Model file for the job. Use its own axes, mm. Face numbers are marked on the shaded views. Round coordinates to 2 decimals unless told otherwise and drop trailing zeros. Write each loop counter-clockwise with the first axis right and the second up, starting at its lowest first coordinate (ties: lowest second). Pieces come first, ordered by that corner, then holes. Notation, with made-up numbers: (38.25, 85.25) - (48.25, 85.25) arc R14 ccw to (48.25, 99.25) - close; hole circle Ø7 at (71.5, 2.25). An arc over 180 degrees is marked (long way). One line per item, written item: value.
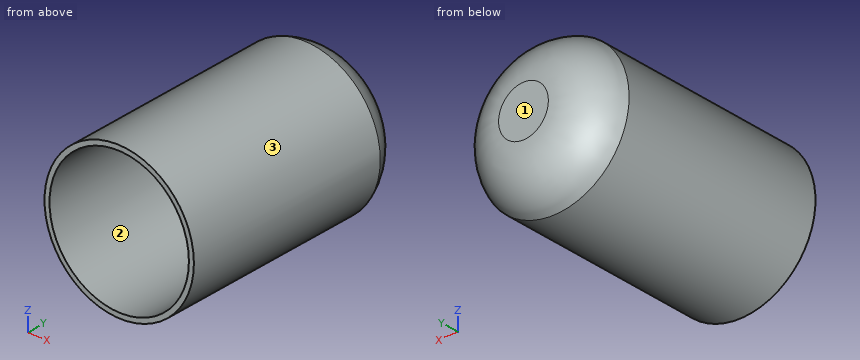
from build123d import *

# Parameters (mm, degrees)
F0_R     = 38.1
F1_DEPTH = 127
F6_T     = -2.54


# Not quite as in the source:
# - a feature of the source that left no trace in its solid (it failed there, or was rolled back) is left out


with BuildPart() as f1:
    # F0 (on Front) → F1 (new body)
    with BuildSketch(Plane.XZ):
        Circle(F0_R)
    extrude(amount=F1_DEPTH)

    # F2 (on Top) → F3 (revolve, cut)
    with BuildSketch(Plane.XY):
        with BuildLine():
            Line((-12.7, 0), (0, 0))
            Line((0, 0), (0, 26.976691559))
            Line((0, 26.976691559), (-68.359054625, 26.976691559))
            Line((-68.359054625, 26.976691559), (-68.359054625, -28.0306376517))
            Line((-68.359054625, -28.0306376517), (-39.5489111543, -28.0306376517))
            ThreePointArc((-39.5489111543, -28.0306376517), (-32.1073483334, -8.2846551837), (-12.7, 0))
        make_face()
    revolve(axis=Axis((0, 13.4883457795, 0), (0, -1, 0)), mode=Mode.SUBTRACT)

    # F6
    f6_openings = [f1.faces().sort_by_distance(p)[0] for p in [
        (0, -127, 0),
    ]]
    offset(amount=F6_T, openings=f6_openings)


solid = f1.part
1. Mould opens along Z. For the marked faces 1, 2 and 3 say: released by +Z, released by -Z, zero draft, split by the parting line, or undercut.
Report:
face 1: zero draft
face 2: undercut
face 3: split by the parting line
2. Band-saw the part on A-A on y = -25.5. Write the cut outline in (x, z), plus the area to 3 significant figures.
Report:
outline: circle Ø76.2 at (0, 0); hole circle Ø71.12 at (0, 0)
area: 588 mm²
3. Drop flat-ended pins along their axis: pin 1 (4 mm diameter, centred on x = -2.5, y = -75, fed in from +Z); pin 2 (6 mm diameter, centred on x = 5, y = -110.5, fed in from -Z); pin 3 (2 mm diameter, centred on x = -4.5, z = 18, fed in from -Y). Give the stop position or say it passes through.
Report:
pin 1: z = 38.1
pin 2: z = -38.05
pin 3: y = -3.53
4. Wall check: probe 1 along Z at (x, y) = (0, -88); probe 2 along Y at (x, z) = (-6.5, 12). Give the ranges that are in metal, low to high. Write a range as [from, to].
Report:
probe 1: [-38.1, -35.56], [35.56, 38.1]
probe 2: [-2.56, -0.02]
